Autodesk Inventor part; units mm, degrees
ref_plane "YZ Plane" through (0, 0, 0) normal (1, 0, 0) x (0, 1, 0)
ref_plane "XZ Plane" through (0, 0, 0) normal (0, 1, 0) x (-1, 0, 0)
ref_plane "XY Plane" through (0, 0, 0) normal (0, 0, 1) x (1, 0, 0)
sketch "Sketch1" plane through (0, 0, 0) normal (1, 0, 0) x (0, 1, 0)
  line L0 (0, 0) -> (16.51, 0)
  line L1 (16.51, 0) -> (16.51, 44.45)
  line L2 (16.51, 44.45) -> (0, 44.45)
  line L3 (0, 44.45) -> (0, 0)
  line L4 (1.27, 44.45) -> (1.27, 0)
  circle A0 centre (8.89, 44.45) radius 7.62
  line L5 (0, 44.45) -> (2.3586, 48.3749)
  circle A1 centre (8.89, 44.45) radius 2.54
  line L6 (8.255, 0) -> (16.51, 8.255)
  dimension "d2" = 15.24
  dimension "d0" = 44.45
  dimension "d1" = 1.27
  dimension "d3" = 7.62
  dimension "d4" = 5.08
  dimension "d5" = 45
extrude "Extrusion1" add sketch "Sketch1" along normal mid plane 31.75 contours L3 L2 L4 L0 | L4 A0 L1 L6 L0 | A0 L2 A1 | L2 A1 A0 | A1 L2 | L2 A1
extrude "Extrusion2" cut sketch "Sketch1" along normal through all both and the other way through all contours A1 L2 | L2 A1
extrude "Extrusion3" cut sketch "Sketch1" along normal mid plane 26.67 contours L4 A0 L1 L6 L0 | A0 L2 A1 | L2 A1 A0 | L2 A1 picked at (9.5237, 43.4833)
properties part number "LegHolderV2"
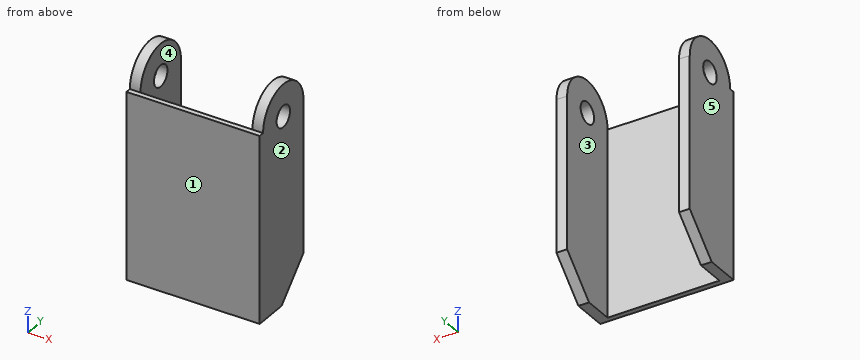
Verification items for the finished model (mm, model axes). Face numbers are marked on the shaded views. A direction names the side the tool comes from. Coordinates: 2 decimals unless noted, no trailing zeros. Write each loop counter-clockwise with the first axis right and the second up, starting at its lowest first coordinate (ties: lowest second). Pieces come first, ordered by that corner, then holes. Notation, with made-up numbers: M 11,37.25 L 49,37.25 A22 ccw 49,48.25 Z; hole C 20.25,7.25 d7. An arc over 180 degrees is marked long. Answer as a JSON object with one key per item and string values. Group by question number.
(1) Cross-section at B-B, the plane z = 32.5. Record the cut outline in (x, y) (3 decimals), and give its area (3 significant figures).
(2) Tool access check on the marked faces 4 and 5. Record the directions out of +Z, -Z, +X, -X, +Y, -Y that give a thin tool (end or side, any length) a straight path to the whole face; none if there is none.
(3) Release check for a two-part mould opening along X. For the marked faces 1, 2 and 3 record: +X half, -X half, draft (parallel to the pull), parting line (faces both ways), or undercut.
(4) Cross-section at D-D, the plane y = 5. Record the cut outline in (x, z) (3 decimals), and give its area (3 significant figures).
(5) Gauge pin test, flat ends, axial feed: pin 1 (12 mm diameter, centred on x = -2, z = 13, fed in from -Y); pin 2 (8 mm diameter, centred on x = 1, z = 29.5, fed in from +Y); pin 3 (4 mm diameter, centred on y = 8.89, z = 44.45, fed in from +X). Record the tip position at first contact, or that the pin passes through.
(6) Material ranges on line 1 (X direction, y = 3.75, z = 42.5) (3 decimals); line 2 (Y direction, x = -13, z = 14.5); line 3 (Z direction, x = -14.3, y = 8.89) (3 decimals), recorded low to high.
(7) Cross-section at A-A, the plane z = 48. Record the cut outline in (x, y) (3 decimals), and give its area (3 significant figures).
(8) Cross-section at C-C, the plane y = 9. Record the cut outline in (x, z) (3 decimals).
Reply:
{
 "1": {"outline": "M -15.875,0 L 15.875,0 L 15.875,16.51 L 13.335,16.51 L 13.335,1.27 L -13.335,1.27 L -13.335,16.51 L -15.875,16.51 Z", "area": "118 mm²"},
 "2": {"face 4": "+Z, -Z, +Y", "face 5": "+Z, -Z, -X, +Y, -Y"},
 "3": {"face 1": "draft", "face 2": "+X half", "face 3": "undercut"},
 "4": {"outline": "M -15.875,0 L -13.335,0 L -13.335,51.002 L -15.875,51.002 Z; M 13.335,0 L 15.875,0 L 15.875,51.002 L 13.335,51.002 Z", "area": "259 mm²"},
 "5": {"pin 1": "y = 0", "pin 2": "y = 1.27", "pin 3": "through"},
 "6": {"line 1": "-15.875 to -13.335, 13.335 to 15.875", "line 2": "0 to 1.27", "line 3": "0.635 to 41.91, 46.99 to 52.07"},
 "7": {"outline": "M -15.875,2.147 L -13.335,2.147 L -13.335,15.633 L -15.875,15.633 Z; M 13.335,2.147 L 15.875,2.147 L 15.875,15.633 L 13.335,15.633 Z", "area": "68.5 mm²"},
 "8": {"outline": "M -15.875,0.745 L -13.335,0.745 L -13.335,41.912 L -15.875,41.912 Z; M -15.875,46.988 L -13.335,46.988 L -13.335,52.069 L -15.875,52.069 Z; M 13.335,0.745 L 15.875,0.745 L 15.875,41.912 L 13.335,41.912 Z; M 13.335,46.988 L 15.875,46.988 L 15.875,52.069 L 13.335,52.069 Z"}
}
